from build123d import *

# Parameters (mm, degrees)
SFAZOWANIE1_SIZE = 1


with BuildPart() as part:
    # Szkic1 → Obrót1 (revolve)
    with BuildSketch(Plane.XY, mode=Mode.PRIVATE) as obr_t1_sk:
        Polygon((-15, -70.098020295), (-15, 29.901979705), (-35, 29.901979705), (-35, 19.901979705), (-30, 19.901979705), (-30, -8.098020295), (-28, -8.098020295), (-28, -23.098020295), (-25, -23.098020295), (-25, -65.098020295), (-22.113248654, -70.098020295), align=None)
    revolve(obr_t1_sk.sketch.rotate(Axis((0, 34.945352564, 0), (0, -1, 0)), 270), axis=Axis((0, 34.945352564, 0), (0, -1, 0)))

    # Sfazowanie1
    sfazowanie1_edges = [part.edges().sort_by_distance(p)[0] for p in [
        (0, 19.901979705, -35),
        (0, 29.901979705, -35),
        (0, 29.901979705, -15),
        (0, -70.098020295, -15),
        (0, -23.098020295, -28),
        (0, -8.098020295, -30),
    ]]
    chamfer(sfazowanie1_edges, length=SFAZOWANIE1_SIZE)


solid = part.part
CAD build for the part. Positions are in the model's coordinates, mm. A direction names the side the tool comes from. Coordinates: 2 decimals unless noted, no trailing zeros. Write each loop counter-clockwise with the first axis right and the second up, starting at its lowest first coordinate (ties: lowest second). Pieces come first, ordered by that corner, then holes. Notation, with made-up numbers: M -0.5,56.25 L 46.5,56.25 A24 ccw 46.5,68.25 Z; hole C 49,6 d3. An arc over 180 degrees is marked long. Answer as a JSON object with one key per item and string values. Group by question number.
1) Mould opens along Z. For faces 1 (the face through (-24, -8.098, -15)), 2 (the face through (27.334, -15.196, -6.07)), 3 (the face through (-0.66, -19.412, -14.985)) say: +Z half, -Z half, draft (parallel to the pull), parting line (faces both ways), or undercut.
2) Wall check: line 1 (X direction, y = -16, z = 0); line 2 (X direction, y = -44, z = 0); line 3 (Z direction, x = -4, y = 16.5). Give the ranges that are in metal, low to high. Write a range as from..to.
3) Saw through at D-D (y = -12.5). Write the cut outline in (x, z).
4) Saw through at C-C (y = -29). Write the cut outline in (x, z), plus the area to 3 significant figures.
5) Pin check, flat tips, straight feed: pin 1 Ø6 at (y, z) = (-14.5, -27) entering from -X; pin 2 Ø10 at (x, y) = (-27, -8.5) entering from +Z; pin 3 Ø12 at (x, z) = (-6, 12) entering from +Y; pin 4 Ø1.5 at (x, y) = (-23.5, -56.5) entering from +Z. Stop position of each tip, or through.
6) Tool access for faces 4 (the face through (8, -23.098, 24)), 5 (the face through (7, 29.902, -15)): list every direction of +Z, -Z, +X, -X, +Y, -Y with a clear straight run to the whole face (end or side of a thin tool).
Values follow:
{
 "1": {"face 1": "draft", "face 2": "parting line", "face 3": "undercut"},
 "2": {"line 1": "x = -28..-15, 15..28", "line 2": "x = -25..-15, 15..25", "line 3": "z = -29.73..-14.46, 14.46..29.73"},
 "3": {"outline": "C 0,0 d56; hole C 0,0 d30"},
 "4": {"outline": "C 0,0 d50; hole C 0,0 d30", "area": "1,260 mm2"},
 "5": {"pin 1": "stops at x = -14.42", "pin 2": "stops at z = 20.18", "pin 3": "stops at y = 29.9", "pin 4": "stops at z = 10.37"},
 "6": {"face 4": "-Y", "face 5": "+Z, -Z, +X, -X, +Y"}
}
